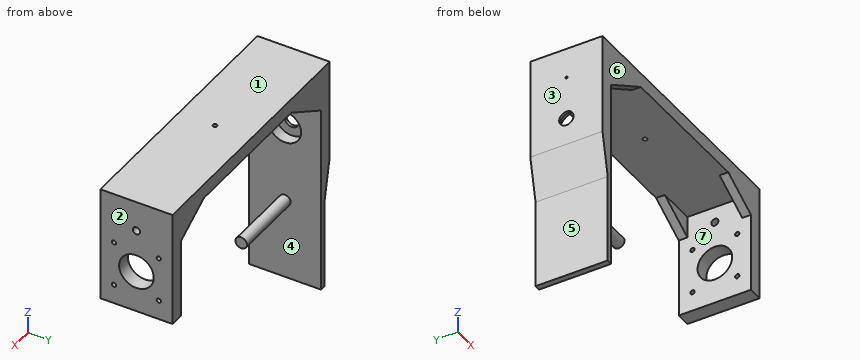
```python
from build123d import *

# Parameters (mm, degrees)
BOSS_EXTRUDE1_DEPTH = 50
SKETCH3_R           = 2.5
SKETCH3_R_2         = 12
SKETCH3_R_3         = 1.5
CUT_EXTRUDE1_DEPTH  = 10
RIB1_REACH          = 129.376
SKETCH4_WALL_W      = 286.752677288
SKETCH4_WALL_H      = 6
MIRROR2_DEPTH       = 6
MIRROR2_START       = 44
MIRROR2_2_DEPTH     = 6
SKETCH5_R           = 11.3
SKETCH5_R_2         = 2.5
CUT_EXTRUDE2_DEPTH  = 8
SKETCH6_R           = 5
SKETCH6_R_2         = 0.75
CUT_EXTRUDE3_DEPTH  = 2
SKETCH8_W           = 4
SKETCH8_H           = 50
BOSS_EXTRUDE2_DEPTH = 91
BOSS_EXTRUDE3_DEPTH = 50
SKETCH11_R          = 1.5
CUT_EXTRUDE4_DEPTH  = 10
SKETCH12_R          = 4.004666462
BOSS_EXTRUDE4_DEPTH = 50


# Read off the part's stored shape, not the designer's step: Mirror2
with BuildPart() as part:
    # Sketch2 → Boss-Extrude1 (new body)
    with BuildSketch(Plane(origin=(0, 0, 0), x_dir=(1, 0, 0), z_dir=(0, 1, 0))):
        Polygon((-83.940042827, 0), (76.059957173, 0), (76.059957173, 70), (86.059957173, 70), (86.059957173, -10), (-93.940042827, -10), (-93.940042827, 60), (-83.940042827, 60), align=None)
    extrude(amount=BOSS_EXTRUDE1_DEPTH)

    # Sketch3 → Cut-Extrude1 (cut)
    with BuildSketch(Plane(origin=(86.059957173, 0, 0), x_dir=(0, 0, -1), z_dir=(1, 0, 0))):
        with Locations((11, 25)):
            Circle(SKETCH3_R)
        with Locations((41, 25)):
            Circle(SKETCH3_R_2)
        with Locations((25.500219356, 40.499780644)):
            Circle(SKETCH3_R_3)
        with Locations((56.499780644, 40.499780644)):
            Circle(SKETCH3_R_3)
        with Locations((56.499780644, 9.500219356)):
            Circle(SKETCH3_R_3)
        with Locations((25.500219356, 9.500219356)):
            Circle(SKETCH3_R_3)
    extrude(amount=-CUT_EXTRUDE1_DEPTH, mode=Mode.SUBTRACT)

    # Sketch4 wall → Rib1 (add, up to next)
    with BuildSketch(Plane(origin=(63.069576117, 50, -7.5), x_dir=(0.86602540378, 0, -0.500000000008), z_dir=(-0.500000000008, 0, -0.86602540378)), mode=Mode.PRIVATE) as rib1_sk1:
        with Locations((0, 3)):
            Rectangle(SKETCH4_WALL_W, SKETCH4_WALL_H)
    rib1_tool1 = extrude(rib1_sk1.sketch, amount=-RIB1_REACH, mode=Mode.PRIVATE) - part.part
    rib1 = rib1_tool1.solids().sort_by_distance((63.069576117, 50, -7.5))[0]
    add(rib1)

    # Mirror1: Rib1 across plane
    add(rib1.mirror(Plane.ZX.offset(25)))

    # Mirror2 outline → Mirror2 (add)
    with BuildSketch(Plane(origin=(0, 0, 0), x_dir=(1, 0, 0), z_dir=(0, 1, 0))):
        Polygon((-83.940042827, 0), (-50.07919506, 0), (-83.940042827, 19.549569573), align=None)
    extrude(amount=MIRROR2_DEPTH)

    # Mirror2 2 outline → Mirror2 2 (add)
    with BuildSketch(Plane(origin=(0, 0, 0), x_dir=(1, 0, 0), z_dir=(0, 1, 0)).offset(MIRROR2_START)):
        Polygon((-83.940042827, 0), (-50.07919506, 0), (-83.940042827, 19.549569573), align=None)
    extrude(amount=MIRROR2_2_DEPTH)

    # Sketch5 → Cut-Extrude2 (cut)
    with BuildSketch(Plane(origin=(-83.940042827, 0, 0), x_dir=(0, 0, -1), z_dir=(1, 0, 0))):
        with Locations((41, 25)):
            Circle(SKETCH5_R)
        with Locations((11, 25)):
            Circle(SKETCH5_R_2)
    extrude(amount=-CUT_EXTRUDE2_DEPTH, mode=Mode.SUBTRACT)

    # Sketch6 → Cut-Extrude3 (cut)
    with BuildSketch(Plane.ZY.offset(93.940042827)):
        with Locations((-41, 25)):
            Circle(SKETCH6_R)
        with Locations((-11, 25)):
            Circle(SKETCH6_R_2)
    extrude(amount=-CUT_EXTRUDE3_DEPTH, mode=Mode.SUBTRACT)

    # Sketch8 → Boss-Extrude2 (add)
    with BuildSketch(Plane(origin=(0, 0, -60), x_dir=(-1, 0, 0), z_dir=(0, 0, -1))):
        with Locations((85.940042827, 25)):
            Rectangle(SKETCH8_W, SKETCH8_H)
    extrude(amount=BOSS_EXTRUDE2_DEPTH)

    # Sketch9 → Boss-Extrude3 (add)
    with BuildSketch(Plane(origin=(0, 50, 0), x_dir=(1, 0, 0), z_dir=(0, 1, 0))):
        Polygon((-87.940042827, 89.393876913), (-93.940042827, 60), (-87.940042827, 60), align=None)
    extrude(amount=-BOSS_EXTRUDE3_DEPTH)

    # Sketch11 → Cut-Extrude4 (cut)
    with BuildSketch(Plane.XY.offset(10)):
        with Locations((-3.940042827, 25)):
            Circle(SKETCH11_R)
    extrude(amount=-CUT_EXTRUDE4_DEPTH, mode=Mode.SUBTRACT)

    # Sketch12 → Boss-Extrude4 (add)
    with BuildSketch(Plane(origin=(-83.940042827, 0, 0), x_dir=(0, 0, -1), z_dir=(1, 0, 0))):
        with Locations(Location((94.840711844, 25, 0), (0, 0, 180))):
            Circle(SKETCH12_R)
    extrude(amount=BOSS_EXTRUDE4_DEPTH)


solid = part.part
```
Model file for the job. Use its own axes, mm. Face numbers are marked on the shaded views. A direction names the side the tool comes from. Give positions to 0.01 mm unless a question says otherwise; leave off trailing zeros. Loops run counter-clockwise (first coordinate to the right, second up) from the corner with the lowest first, then second, coordinate; pieces in that order, holes last. Notation, with made-up numbers: M -19,-16.5 L 40,-16.5 A11 ccw 40,-4.5 Z; hole C -33,70.5 d9. An arc over 180 degrees is marked long. Use one line per item in the form item = value.
Item 1: Slice it at D-D on z = -138.5. List the corners of the cut face in (x, y).
Filled in:
outline = M -87.94,0 L -83.94,0 L -83.94,50 L -87.94,50 Z
Item 2: Slice it at A-A on z = -41. List the corners of the cut face in (x, y), and give its area (3 significant figures).
Filled in:
outline = M -93.94,0 L -83.94,0 L -83.94,13.7 L -91.94,13.7 L -91.94,20 L -93.94,20 Z; M -93.94,30 L -91.94,30 L -91.94,36.3 L -83.94,36.3 L -83.94,50 L -93.94,50 Z; M 76.06,0 L 86.06,0 L 86.06,13 L 76.06,13 Z; M 76.06,37 L 86.06,37 L 86.06,50 L 76.06,50 Z
area = 559 mm^2
Item 3: Two-plate mould, pull along X, no slides. Class the marked faces 1, 2, 3 and 4: released by +X, released by -X, zero draft, split by the parting line, or undercut.
Filled in:
face_1 = zero draft
face_2 = released by +X
face_3 = released by -X
face_4 = undercut
Item 4: Flat gauge pins, fed straight in: pin 1 Ø2.5 at (y, z) = (9.5, -25.5) entering from +X; pin 2 Ø4 at (y, z) = (25, -11) entering from -X; pin 3 Ø8 at (x, y) = (80.5, 17.5) entering from -Z; pin 4 Ø2.5 at (y, z) = (24.5, -96.5) entering from +X. Where does each tip first touch, or does it go through?
Filled in:
pin_1 = -83.94
pin_2 = -93.94
pin_3 = -70
pin_4 = -33.94
Item 5: Drill centre lines: L1, parallel to Y at x = -93.05, z = -41; L2, parallel to X at y = 29.5, z = -57.5; L3, parallel to Y at x = 79, z = -41. Where is each one in solid material? Low to high.
Filled in:
L1 = 0 to 20, 30 to 50
L2 = -93.94 to -83.94, 76.06 to 86.06
L3 = 0 to 13, 37 to 50
Item 6: Slice it at C-C on z = -62.5. List the corners of the cut face in (x, y).
Filled in:
outline = M -93.43,0 L -83.94,0 L -83.94,50 L -93.43,50 Z; M 76.06,0 L 86.06,0 L 86.06,50 L 76.06,50 Z
Item 7: Slice it at B-B on x = -37. List the corners of the cut face in (y, z), and give its area (3 significant figures).
Filled in:
outline = M 0,0 L 50,0 L 50,10 L 0,10 Z; C 25,-94.84 d8.01
area = 550 mm^2
Item 8: Which spindle directions (+Z, -Z, +X, -X, +Y, -Y) get a long thin tool onto all of the face, cutting with end or side? Do the marked faces 5, 6 and 7. Say none if no direction does.
Filled in:
face_5 = -Z, -X, +Y, -Y
face_6 = +Z, -Z, +X, -X, -Y
face_7 = -Z
